CAD build for the part. Positions are in the model's coordinates, mm. Face numbers are marked on the shaded views. A direction names the side the tool comes from. Give positions to 0.01 mm unless a question says otherwise; leave off trailing zeros. Loops run counter-clockwise (first coordinate to the right, second up) from the corner with the lowest first, then second, coordinate; pieces in that order, holes last. Notation, with made-up numbers: (11.25, 56.5) -> (47.25, 56.5) arc R14 ccw to (47.25, 70.5) -> close; hole circle Ø4 at (-14, 70.25). An arc over 180 degrees is marked (long way). Use one line per item in the form item = value.
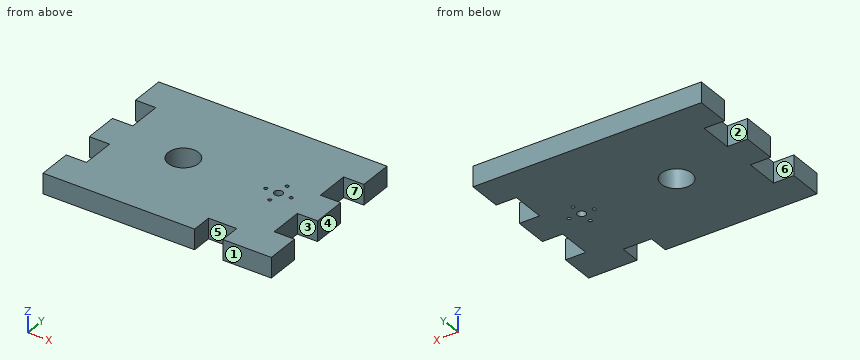
```python
from build123d import *

# Parameters (mm, degrees)
SKETCH1_W           = 171.45
SKETCH1_H           = 127
BOSS_EXTRUDE1_DEPTH = 15.24
SKETCH5_W           = 15.24
SKETCH5_H           = 25.4
CUT_EXTRUDE1_DEPTH  = 15.24
SKETCH11_R          = 11.43
CUT_EXTRUDE3_DEPTH  = 15.24
SKETCH12_R          = 3.175
SKETCH12_R_2        = 1.27
CUT_EXTRUDE4_DEPTH  = 15.24
SKETCH7_W           = 21.166666666
SKETCH7_H           = 15.24
CUT_EXTRUDE5_DEPTH  = 15.24


with BuildPart() as part:
    # Sketch1 → Boss-Extrude1 (new body)
    with BuildSketch(Plane.XY):
        with Locations((85.725, 63.5)):
            Rectangle(SKETCH1_W, SKETCH1_H)
    extrude(amount=BOSS_EXTRUDE1_DEPTH)

    # Sketch5 → Cut-Extrude1 (cut)
    with BuildSketch(Plane.XY.offset(15.24)):
        with Locations((7.62, 88.9)):
            Rectangle(SKETCH5_W, SKETCH5_H)
        with Locations((7.62, 38.1)):
            Rectangle(SKETCH5_W, SKETCH5_H)
        with Locations((163.83, 88.9)):
            Rectangle(SKETCH5_W, SKETCH5_H)
        with Locations((163.83, 38.1)):
            Rectangle(SKETCH5_W, SKETCH5_H)
    extrude(amount=-CUT_EXTRUDE1_DEPTH, mode=Mode.SUBTRACT)

    # Sketch11 → Cut-Extrude3 (cut)
    with BuildSketch(Plane.XY.offset(15.24)):
        with Locations((61.976, 63.5)):
            Circle(SKETCH11_R)
    extrude(amount=-CUT_EXTRUDE3_DEPTH, mode=Mode.SUBTRACT)

    # Sketch12 → Cut-Extrude4 (cut)
    with BuildSketch(Plane.XY.offset(15.24)):
        with Locations((133.35, 63.5)):
            Circle(SKETCH12_R)
        with Locations((133.35, 73.025)):
            Circle(SKETCH12_R_2)
        with Locations((142.875, 63.5)):
            Circle(SKETCH12_R_2)
        with Locations((133.35, 53.975)):
            Circle(SKETCH12_R_2)
        with Locations((123.825, 63.5)):
            Circle(SKETCH12_R_2)
    extrude(amount=-CUT_EXTRUDE4_DEPTH, mode=Mode.SUBTRACT)

    # Sketch7 → Cut-Extrude5 (cut)
    with BuildSketch(Plane.XY.offset(15.24)):
        with Locations((124.46, 7.62)):
            Rectangle(SKETCH7_W, SKETCH7_H)
    extrude(amount=-CUT_EXTRUDE5_DEPTH, mode=Mode.SUBTRACT)


solid = part.part
```
1. Cut at A-A, the plane z = 9.25. State how many separate pieces and enclosed holes the cut face has, then the cut area to 3 significant figures.
Result sheet:
separate_pieces = 1
enclosed_holes = 6
area = 19,400 mm^2
2. Cut at C-C, the plane y = 48. Write the cut outline in (x, z), then the cut area to 3 significant figures.
Result sheet:
outline = (15.24, 0) -> (156.21, 0) -> (156.21, 15.24) -> (15.24, 15.24) -> close
area = 2,150 mm^2
3. Tool access for the marked faces 5, 6 and 7: list every direction of +Z, -Z, +X, -X, +Y, -Y with a clear straight run to the whole face (end or side of a thin tool).
Result sheet:
face_5 = +Z, -Z, -Y
face_6 = +Z, -Z, -X
face_7 = +Z, -Z, +X
4. Cut at B-B, the plane y = 69.5. Write the cut outline in (x, z), then the cut area to 3 significant figures.
Result sheet:
outline = (0, 0) -> (52.25, 0) -> (52.25, 15.24) -> (0, 15.24) -> close; (71.7, 0) -> (171.45, 0) -> (171.45, 15.24) -> (71.7, 15.24) -> close
area = 2,320 mm^2
5. Mould opens along Y. For the marked faces 1, 2, 3 and 4 say: pulls with the +Y half, pulls with the -Y half, needs draft (parallel to the pull), parting line crosses it, or undercut.
Result sheet:
face_1 = pulls with the -Y half
face_2 = undercut
face_3 = undercut
face_4 = needs draft
6. Drill centre lines: line 1 (Y direction, x = 163.5, z = 14.25); line 2 (Y direction, x = 133.35, z = 7) (3 decimals); line 3 (X direction, y = 65, z = 3.75). Where is each one in solid material? Low to high.
Result sheet:
line_1 = 0 to 25.4, 50.8 to 76.2, 101.6 to 127
line_2 = 15.24 to 52.705, 55.245 to 60.325, 66.675 to 71.755, 74.295 to 127
line_3 = 0 to 50.64, 73.31 to 130.55, 136.15 to 171.45
7. Drop flat-ended pins along their axis: P1, Ø7.5, axis at x = 127, z = 9, coming from the -Y side; P2, Ø5.5, axis at x = 133.35, y = 63.5, coming from the +Z side; P3, Ø3, axis at y = 90.5, z = 6.5, coming from the +X side; P4, Ø5, axis at y = 79.5, z = 4, coming from the -X side. Give the stop position or say it passes through.
Result sheet:
P1 = 15.24
P2 = through
P3 = 156.21
P4 = 15.24
